Verification items for this drawing (mm, ordinates from the low corner). Give positions to 0.01 mm unless a question says otherwise; leave off trailing zeros. Order: outer loops, then holes, each group sorted by start corner. A loop starts at its lowest first (then second) coordinate and runs counter-clockwise, first axis right, second up.
(1) Sectioned sample at C-C on y = 52. Record the cut outline in (x, z).
(2) Scan lines: L1, parallel to Y at x = 20, z = 1.8; L2, parallel to Y at x = 89.25, z = 2.3; L3, parallel to X at y = 40, z = 2. Record each from-to range of solid material in increasing order.
(3) Gauge pin test, flat end, axial feed: pin 1 (1.5 mm diameter, centred on y = 11, z = 2, fed in from -X). Record the tip position at first contact, or that the pin passes through.
(4) Sectioned sample at A-A on y = 40. Record the cut outline in (x, z), plus the area to 3 significant figures.
(5) Sectioned sample at D-D on x = 89.25. Record the cut outline in (y, z), plus the area to 3 significant figures.
(6) Sectioned sample at B-B on x = 70. Record the cut outline in (y, z), plus the area to 3 significant figures.
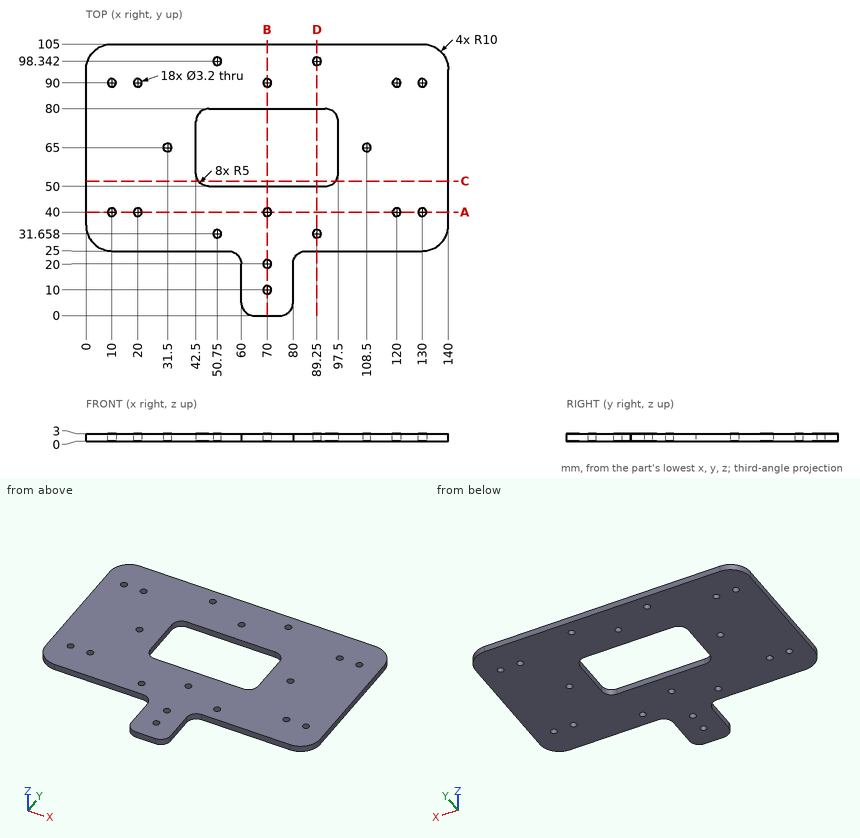
Ans:
1. outline: (0, 0) - (43.5, 0) - (43.5, 3) - (0, 3) - close; (96.5, 0) - (140, 0) - (140, 3) - (96.5, 3) - close
2. L1: y = 25 to 38.4, 41.6 to 88.4, 91.6 to 105
2. L2: y = 25 to 30.06, 33.26 to 50, 80 to 96.74, 99.94 to 105
2. L3: x = 0 to 8.4, 11.6 to 18.4, 21.6 to 68.4, 71.6 to 118.4, 121.6 to 128.4, 131.6 to 140
3. pin 1: stops at x = 60
4. outline: (0, 0) - (8.4, 0) - (8.4, 3) - (0, 3) - close; (11.6, 0) - (18.4, 0) - (18.4, 3) - (11.6, 3) - close; (21.6, 0) - (68.4, 0) - (68.4, 3) - (21.6, 3) - close; (71.6, 0) - (118.4, 0) - (118.4, 3) - (71.6, 3) - close; (121.6, 0) - (128.4, 0) - (128.4, 3) - (121.6, 3) - close; (131.6, 0) - (140, 0) - (140, 3) - (131.6, 3) - close
4. area: 372 mm2
5. outline: (25, 0) - (30.06, 0) - (30.06, 3) - (25, 3) - close; (33.26, 0) - (50, 0) - (50, 3) - (33.26, 3) - close; (80, 0) - (96.74, 0) - (96.74, 3) - (80, 3) - close; (99.94, 0) - (105, 0) - (105, 3) - (99.94, 3) - close
5. area: 131 mm2
6. outline: (0, 0) - (8.4, 0) - (8.4, 3) - (0, 3) - close; (11.6, 0) - (18.4, 0) - (18.4, 3) - (11.6, 3) - close; (21.6, 0) - (38.4, 0) - (38.4, 3) - (21.6, 3) - close; (41.6, 0) - (50, 0) - (50, 3) - (41.6, 3) - close; (80, 0) - (88.4, 0) - (88.4, 3) - (80, 3) - close; (91.6, 0) - (105, 0) - (105, 3) - (91.6, 3) - close
6. area: 187 mm2
